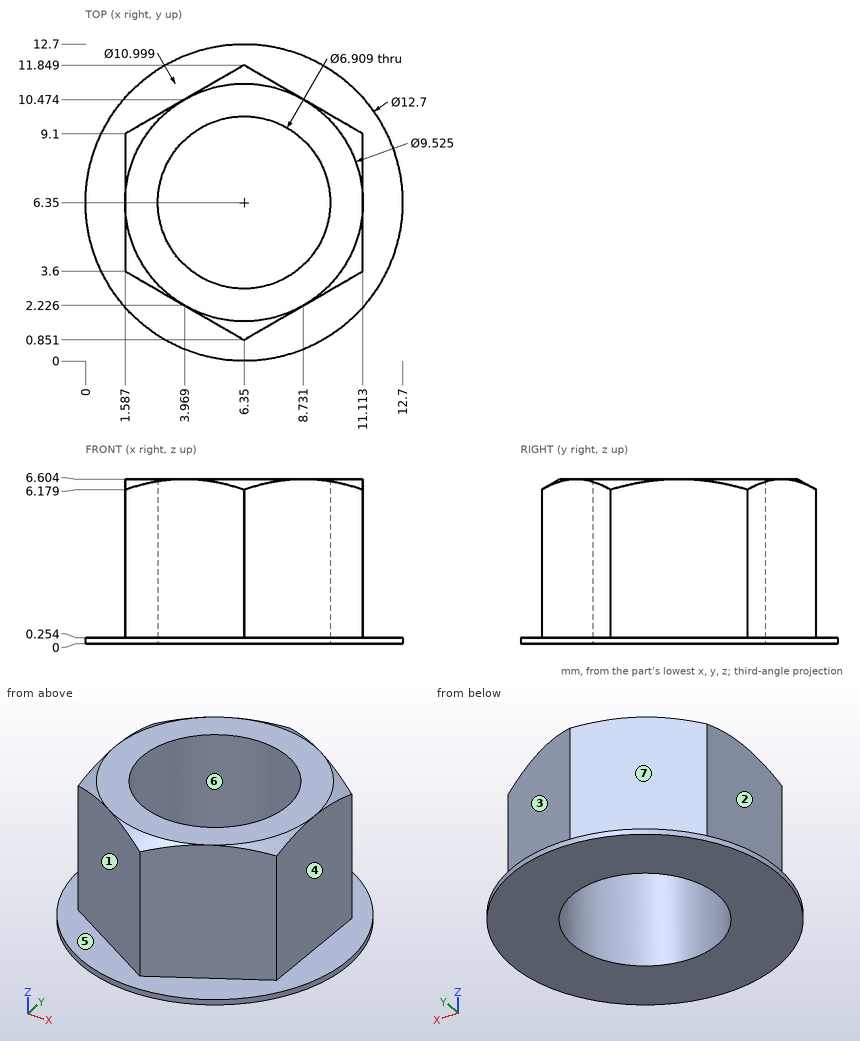
The figure shows three views and two pictorial views of one solid part (mm, origin at its lowest corner). Answer the questions. A direction names the side the tool comes from. Give positions to 0.01 mm unless a question says otherwise; leave off trailing zeros. Use one line per item in the form item = value. Start each with the question number.
1) The mould has two halves that part along X. Classify the marked faces 4, 5, 6 and 7: pulls with the +X half, pulls with the -X half, needs draft (parallel to the pull), parting line crosses it, or undercut.
2) Flat-ended cylindrical pins translate along their axes: pin 1 Ø1.6 at (y, z) = (6, 2) entering from -X; pin 2 Ø1.5 at (x, z) = (8, 5.5) entering from -Y; pin 3 Ø1.5 at (x, y) = (4.5, 5) entering from -Z; pin 4 Ø1 at (y, z) = (4.5, 2) entering from +X. Find the tip coordinate at first contact, or state that the pin passes through.
3) Consider line 1 along X through (y, z) = (6.5, 1.75); line 2 along Y through (x, z) = (6.25, 3) (1 decimal); line 3 along X through (y, z) = (7.25, 1.75) (1 decimal). Determine where each line is inside the solid, lowest interval first. Write a range as from..to.
4) A tool of negligible diameter and unlimited length cuts with its end or side. For the marked faces 1, 2 and 3, from which of +Z, -Z, +X, -X, +Y, -Y can it reach the whole face along a straight path? Write none if from no direction.
Geometry results:
q1.face_4 = pulls with the +X half
q1.face_5 = needs draft
q1.face_6 = undercut
q1.face_7 = pulls with the -X half
q2.pin_1 = 1.59
q2.pin_2 = 1.37
q2.pin_3 = through
q2.pin_4 = 11.11
q3.line_1 = 1.59..2.9, 9.8..11.11
q3.line_2 = 0.9..2.9, 9.8..11.8
q3.line_3 = 1.6..3, 9.7..11.1
q4.face_1 = +Z, -X, -Y
q4.face_2 = +Z, -X, +Y, -Y
q4.face_3 = +Z, +X, +Y
